Read the model definition and answer for the solid it produces. Units are mm, in the model's axes. Round coordinates to 2 decimals unless told otherwise and drop trailing zeros. Order: outer loops, then holes, each group sorted by start corner. A loop starts at its lowest first (then second) coordinate and runs counter-clockwise, first axis right, second up. Notation, with made-up numbers: M 76,65.5 L 84,65.5 A22 ccw 84,80.5 Z; hole C -30.75,14.25 d11. An arc over 180 degrees is marked long. Answer as CSV lines item,"result".
```python
from build123d import *

# Parameters (mm, degrees)
SKETCH3_R                = 63.5
BOSS_EXTRUDE1_DEPTH      = 2.54
CUT_EXTRUDE1_REACH       = 91.838
SKETCH4_R                = 7.9375
FILLET1_R                = 2.54
CIRPATTERN1_COUNT        = 4
FILLET1_OF_CIRPATTERN1_R = 2.54


with BuildPart() as part:
    # Sketch3 → Boss-Extrude1 (new body)
    with BuildSketch(Plane(origin=(0, 0, 0), x_dir=(1, 0, 0), z_dir=(0, 1, 0))):
        with Locations(Location((0, 0, 0), (0, 0, 270))):
            Circle(SKETCH3_R)
    extrude(amount=BOSS_EXTRUDE1_DEPTH)

    # Sketch4 → Cut-Extrude1 (cut, up to next)
    with BuildSketch(Plane(origin=(0, 2.54, 0), x_dir=(1, 0, 0), z_dir=(0, 1, 0)), mode=Mode.PRIVATE) as cut_extrude1_sk1:
        with Locations((0, 63.5)):
            Circle(SKETCH4_R)
    cut_extrude1_tool1 = extrude(cut_extrude1_sk1.sketch, amount=-CUT_EXTRUDE1_REACH, mode=Mode.PRIVATE) & part.part
    cut_extrude1 = cut_extrude1_tool1.solids().sort_by_distance((0, 2.54, -63.5))[0]
    add(cut_extrude1, mode=Mode.SUBTRACT)

    # Fillet1
    fillet1_edges = [part.edges().sort_by_distance(p)[0] for p in [
        (7.921981901, 1.27, -63.00390625),
        (-7.921981901, 1.27, -63.00390625),
    ]]
    fillet(fillet1_edges, radius=FILLET1_R)

    # CirPattern1: Cut-Extrude1 ×4 about axis
    cirpattern1_axis = Axis((0, 0, 0), (0, 1, 0))
    for i in range(1, CIRPATTERN1_COUNT):
        add(cut_extrude1.rotate(cirpattern1_axis, i * 360 / CIRPATTERN1_COUNT), mode=Mode.SUBTRACT)

    # Fillet1 of CirPattern1
    fillet1_of_cirpattern1_edges = [part.edges().sort_by_distance(p)[0] for p in [
        (-63.00390625, 1.27, -7.921981901),
        (-63.00390625, 1.27, 7.921981901),
        (-7.921981901, 1.27, 63.00390625),
        (7.921981901, 1.27, 63.00390625),
        (63.00390625, 1.27, 7.921981901),
        (63.00390625, 1.27, -7.921981901),
    ]]
    fillet(fillet1_of_cirpattern1_edges, radius=FILLET1_OF_CIRPATTERN1_R)


solid = part.part
```
Item 1: A cutting plane is placed at A-A, the plane z = 0. Determine the outline of the cut face in (x, y), and give its area (3 significant figures).
Ans:
outline,"M -55.56,0 L 55.56,0 L 55.56,2.54 L -55.56,2.54 Z"
area,"282 mm2"
Item 2: A cutting plane is placed at B-B, the plane x = 46.5. Determine the outline of the cut face in (y, z).
Ans:
outline,"M 0,-43.24 L 2.54,-43.24 L 2.54,43.24 L 0,43.24 Z"
Item 3: A flat-ended cylindrical pin translates along its axis: pin 1 (2 mm diameter, centred on x = 1, z = 7, fed in from -Y). Find the tip coordinate at first contact, or state that the pin passes through.
Ans:
pin 1,"y = 0"
Item 4: Determine the mould class of faces 1 (the face through (45.3, 1.3, -44.5)), 2 (the face through (0.138, 1.288, 55.564)), 3 (the face through (1, 0, -1)), 4 (the face through (-44.5, 1.3, -45.3)) for opening direction X: +X half, -X half, draft (parallel to the pull), parting line (faces both ways), or undercut.
Ans:
face 1,"+X half"
face 2,"undercut"
face 3,"draft"
face 4,"-X half"
Item 5: Find the intervals of material crossed by probe 1 along X at (y, z) = (0.4, 0.5); probe 2 along Z at (x, y) = (44, 0.5); probe 3 along X at (y, z) = (0.6, -53.5), in increasing order. Write a range as [from, to].
Ans:
probe 1,"[-55.58, 55.58]"
probe 2,"[-45.78, 45.78]"
probe 3,"[-34.21, 34.21]"
